Source: CAD feature listing. Evaluate the final solid. Frame: model axes, mm. A direction names the side the tool comes from. Coordinates: 2 decimals unless noted, no trailing zeros. Loops run counter-clockwise (first coordinate to the right, second up) from the corner with the lowest first, then second, coordinate; pieces in that order, holes last. Notation, with made-up numbers: (-1.5, 51) -> (54.5, 51) arc R16 cw to (54.5, 72) -> close; hole circle Ø8 at (38, 83). An arc over 180 degrees is marked (long way). Answer as CSV lines item,"result".
from build123d import *

# Parameters (mm, degrees)
SKETCH1_R           = 1.7
SKETCH1_R_2         = 7.6
BOSS_EXTRUDE1_DEPTH = 8.5
SKETCH1_4_W         = 30
SKETCH1_4_H         = 10
SKETCH1_4_R         = 1.7
BOSS_EXTRUDE2_DEPTH = 15
BOSS_EXTRUDE3_START = 15
SKETCH1_5_R         = 6
SKETCH1_5_W         = 30
SKETCH1_5_H         = 10
SKETCH1_5_R_2       = 1.7
SKETCH1_5_R_3       = 3.2
BOSS_EXTRUDE3_DEPTH = 3
BOSS_EXTRUDE4_START = 18
SKETCH1_6_R         = 6
SKETCH1_6_W         = 30
SKETCH1_6_H         = 10
SKETCH1_6_R_2       = 1.7
BOSS_EXTRUDE4_DEPTH = 2


with BuildPart() as part:
    # Sketch1 → Boss-Extrude1 (new body)
    with BuildSketch(Plane.YZ):
        with BuildLine():
            ThreePointArc((15, 0), (0, 15), (-15, 0))
            Line((-15, 0), (-15, -25.2))
            Line((-15, -25.2), (15, -25.2))
            Line((15, -25.2), (15, 0))
        make_face()
        with Locations(Location((-10.5, -10.7, 0), (0, 0, 270))):
            Circle(SKETCH1_R, mode=Mode.SUBTRACT)
        with Locations(Location((10.5, -10.7, 0), (0, 0, 270))):
            Circle(SKETCH1_R, mode=Mode.SUBTRACT)
        with Locations(Location((0, 0, 0), (0, 0, 270))):
            Circle(SKETCH1_R_2, mode=Mode.SUBTRACT)
        with Locations(Location((7.5, -20.2, 0), (0, 0, 270))):
            Circle(SKETCH1_R, mode=Mode.SUBTRACT)
        with Locations(Location((-7.5, -20.2, 0), (0, 0, 270))):
            Circle(SKETCH1_R, mode=Mode.SUBTRACT)
    extrude(amount=BOSS_EXTRUDE1_DEPTH)

    # Sketch1<4> → Boss-Extrude2 (add)
    with BuildSketch(Plane.YZ):
        with Locations((0, -20.2)):
            Rectangle(SKETCH1_4_W, SKETCH1_4_H)
        with Locations(Location((-7.5, -20.2, 0), (0, 0, 270))):
            Circle(SKETCH1_4_R, mode=Mode.SUBTRACT)
        with Locations(Location((7.5, -20.2, 0), (0, 0, 270))):
            Circle(SKETCH1_4_R, mode=Mode.SUBTRACT)
    extrude(amount=BOSS_EXTRUDE2_DEPTH)

    # Sketch1<5> → Boss-Extrude3 (add)
    # profile 1 of 4: a face of its own
    with BuildSketch(Plane.YZ.offset(BOSS_EXTRUDE3_START)):
        Polygon((15, -25.2), (-15, -25.2), (-15, -80.2), (-10, -85.2), (10, -85.2), (15, -80.2), align=None)
        with Locations((0, -73.2)):
            Circle(SKETCH1_5_R, mode=Mode.SUBTRACT)
        with Locations((0, -37.2)):
            Circle(SKETCH1_5_R, mode=Mode.SUBTRACT)
    # profile 2 of 4: a face of its own
    with BuildSketch(Plane.YZ.offset(BOSS_EXTRUDE3_START)):
        with Locations((0, -20.2)):
            Rectangle(SKETCH1_5_W, SKETCH1_5_H)
        with Locations(Location((-7.5, -20.2, 0), (0, 0, 270))):
            Circle(SKETCH1_5_R_2, mode=Mode.SUBTRACT)
        with Locations(Location((7.5, -20.2, 0), (0, 0, 270))):
            Circle(SKETCH1_5_R_2, mode=Mode.SUBTRACT)
    # profile 3 of 4: a face of its own
    with BuildSketch(Plane.YZ.offset(BOSS_EXTRUDE3_START)):
        with Locations((0, -37.2)):
            Circle(SKETCH1_5_R)
        with Locations(Location((0, -37.2, 0), (0, 0, 270))):
            Circle(SKETCH1_5_R_3, mode=Mode.SUBTRACT)
    # profile 4 of 4: a face of its own
    with BuildSketch(Plane.YZ.offset(BOSS_EXTRUDE3_START)):
        with Locations((0, -73.2)):
            Circle(SKETCH1_5_R)
        with Locations(Location((0, -73.2, 0), (0, 0, 270))):
            Circle(SKETCH1_5_R_3, mode=Mode.SUBTRACT)
    extrude(amount=BOSS_EXTRUDE3_DEPTH)

    # Sketch1<6> → Boss-Extrude4 (add)
    # profile 1 of 2: a face of its own
    with BuildSketch(Plane.YZ.offset(BOSS_EXTRUDE4_START)):
        Polygon((15, -25.2), (-15, -25.2), (-15, -80.2), (-10, -85.2), (10, -85.2), (15, -80.2), align=None)
        with Locations(Location((0, -73.2, 0), (0, 0, 270))):
            Circle(SKETCH1_6_R, mode=Mode.SUBTRACT)
        with Locations(Location((0, -37.2, 0), (0, 0, 270))):
            Circle(SKETCH1_6_R, mode=Mode.SUBTRACT)
    # profile 2 of 2: a face of its own
    with BuildSketch(Plane.YZ.offset(BOSS_EXTRUDE4_START)):
        with Locations((0, -20.2)):
            Rectangle(SKETCH1_6_W, SKETCH1_6_H)
        with Locations(Location((-7.5, -20.2, 0), (0, 0, 270))):
            Circle(SKETCH1_6_R_2, mode=Mode.SUBTRACT)
        with Locations(Location((7.5, -20.2, 0), (0, 0, 270))):
            Circle(SKETCH1_6_R_2, mode=Mode.SUBTRACT)
    extrude(amount=BOSS_EXTRUDE4_DEPTH)


solid = part.part
(1) Cut plane C-C (y = 2). Return the cut outline in (x, z).
Computed values:
outline,"(0, -25.2) -> (15, -25.2) -> (15, -34.7) -> (18, -34.7) -> (18, -31.54) -> (20, -31.54) -> (20, -15.2) -> (8.5, -15.2) -> (8.5, -7.33) -> (0, -7.33) -> close; (0, 7.33) -> (8.5, 7.33) -> (8.5, 14.87) -> (0, 14.87) -> close; (15, -85.2) -> (20, -85.2) -> (20, -78.86) -> (18, -78.86) -> (18, -75.7) -> (15, -75.7) -> close; (15, -70.7) -> (18, -70.7) -> (18, -67.54) -> (20, -67.54) -> (20, -42.86) -> (18, -42.86) -> (18, -39.7) -> (15, -39.7) -> close"
(2) Material intervals for L1, parallel to Y at x = 3, z = -10.7; L2, parallel to Y at x = 19.4, z = -73.2; L3, parallel to Z at x = 8, y = 6.75, sorted ascending. Write a range as [from, to].
Computed values:
L1,"[-15, -12.2], [-8.8, 8.8], [12.2, 15]"
L2,"[-15, -6], [6, 15]"
L3,"[-25.2, -21.73], [-18.67, -3.49], [3.49, 13.4]"
(3) Draft query along Y for faces 1 (the cylindrical face through (4.19, -2.91, -7.02)), 2 (the flat face through (8.5, 6, -7)), 3 (the flat face through (16, -15, -34)), 4 (the flat face through (18, 3, -40)). Return one class per face: released by +Y, released by -Y, zero draft, split by the parting line, or undercut.
Computed values:
face 1,"undercut"
face 2,"zero draft"
face 3,"released by -Y"
face 4,"undercut"
(4) Access query for faces 5 (the flat face through (15, 0, -55)), 6 (the flat face through (14, 0, -15.2)), 7 (the cylindrical face through (18.986, 1.802, -78.923)), 8 (the flat face through (17.5, 12.5, -82.7)). Directions: +Z, -Z, +X, -X, +Y, -Y. A direction counts if a zero-diameter tool reaches every point of the face in a straight line with its end or side. Return the directions, or none.
Computed values:
face 5,"-Z, -X, +Y, -Y"
face 6,"+Z, +X, +Y, -Y"
face 7,"+X"
face 8,"-Z, +X, -X, +Y"
(5) Cut plane D-D (z = -10.7). Return the cut outline in (x, y), then the cut area to 3 significant figures.
Computed values:
outline,"(0, -15) -> (8.5, -15) -> (8.5, -12.2) -> (0, -12.2) -> close; (0, -8.8) -> (8.5, -8.8) -> (8.5, 8.8) -> (0, 8.8) -> close; (0, 12.2) -> (8.5, 12.2) -> (8.5, 15) -> (0, 15) -> close"
area,"197 mm^2"
(6) Cut plane A-A (z = -37.2). Return the cut outline in (x, y), then the cut area to 3 significant figures.
Computed values:
outline,"(15, -15) -> (20, -15) -> (20, -6) -> (18, -6) -> (18, -3.2) -> (15, -3.2) -> close; (15, 3.2) -> (18, 3.2) -> (18, 6) -> (20, 6) -> (20, 15) -> (15, 15) -> close"
area,"107 mm^2"
(7) Pin query (flat end, axial travel): pin 1 Ø6 at (x, y) = (14, 4.5) entering from +Z; pin 2 Ø7.5 at (y, z) = (0, -73.2) entering from -X; pin 3 Ø3.5 at (y, z) = (1.5, -38) entering from +X. Return the tip coordinate at first contact, or that it passes through.
Computed values:
pin 1,"z = -15.2"
pin 2,"x = 15"
pin 3,"x = 18"
(8) Cut plane B-B (x = 7.5). Return the cut outline in (y, z), then the cut area to 3 significant figures.
Computed values:
outline,"(-15, -25.2) -> (15, -25.2) -> (15, 0) arc R15 ccw to (-15, 0) -> close; hole circle Ø3.4 at (-10.5, -10.7); hole circle Ø3.4 at (-7.5, -20.2); hole circle Ø15.2 at (0, 0); hole circle Ø3.4 at (7.5, -20.2); hole circle Ø3.4 at (10.5, -10.7)"
area,"892 mm^2"
